Work out the finished part from the listing and answer in its coordinate system (mm). Face numbers are marked on the shaded views. A direction names the side the tool comes from. Round coordinates to 2 decimals unless told otherwise and drop trailing zeros. Write each loop counter-clockwise with the first axis right and the second up, starting at its lowest first coordinate (ties: lowest second). Pieces come first, ordered by that corner, then holes. Notation, with made-up numbers: M -18.75,17 L 37.25,17 A19 cw 37.25,49 Z; hole C 42.25,64.5 d2. An arc over 180 degrees is marked long. One line per item, written item: value. Start each with the question number.
Q1. A tool of negligible diameter and unlimited length cuts with its end or side. For the marked faces 1, 2, 3 and 4, from which of +Z, -Z, +X, -X, +Y, -Y can it reach the whole face along a straight path? Write none if from no direction.
Q2. Find section C-C (x = 15). Write down the section's boundary in (y, z).
Q3. The mould has two halves that part along X. Classify the marked faces 5, 6, 7 and 8: released by +X, released by -X, zero draft, split by the parting line, or undercut.
Q4. Find section A-A (z = 0). Write down the section's boundary in (x, y), and give its area (4 significant figures).
Q5. Find section D-D (z = -12.5). Write down the section's boundary in (x, y), and give its area (3 significant figures).
Q6. Given pin 1 Ø1 at (y, z) = (4, -18.5) entering from +X; pin 2 Ø1 at (y, z) = (8.5, -14) entering from -X; pin 3 Ø0.6 at (x, y) = (7.5, 2) entering from +Z, each flat-ended and moving along its own axis, determine where each tip first touches the part or whether it passes through.
Q7. Consider probe 1 along X at (y, z) = (1.8, 0); probe 2 along Z at (x, y) = (14.25, 1.5); probe 3 along Y at (x, z) = (3.25, -3). Determine where each line is inside the solid, lowest interval first.
Q8. Find section B-B (y = 4.25). Write down the section's boundary in (x, z).
from build123d import *

# Parameters (mm, degrees)
MAIN_BODY_DEPTH                           = 10
SKETCH1_3_R                               = 1.6
CONNECTOR_BODY_DEPTH                      = 5
DULLING_FILLET_START                      = 5
DULLING_FILLET_DEPTH                      = 6
CUT_EXTRUDE1_DEPTH                        = 45.806187552
FILLET1_R                                 = 2
FILLET2_R                                 = 0.5
ELEPHANTSFOOT_COMPENSATION_LEFT_CONF_SIZE = 0.5


with BuildPart() as part:
    # complete_sketch → main_body (new body)
    with BuildSketch(Plane(origin=(0, 0, 0), x_dir=(1, 0, 0), z_dir=(0, 1, 0))):
        with BuildLine():
            ThreePointArc((-2.5, 8.291561976), (-2.925728922, 5.40481063), (-4.166666667, 2.763853992))
            ThreePointArc((-4.166666667, 2.763853992), (-1.24767584, 4.841828683), (2.312045751, 4.433333333))
            ThreePointArc((2.312045751, 4.433333333), (4.555661111, 3.587465144), (6.936137254, 3.3))
            Line((6.936137254, 3.3), (8.063862746, 3.3))
            ThreePointArc((8.063862746, 3.3), (10.444338889, 3.587465144), (12.687954249, 4.433333333))
            ThreePointArc((12.687954249, 4.433333333), (16.605433979, 4.735248857), (19.531538935, 2.113091309))
            Line((19.531538935, 2.113091309), (3.218923361, 37.095608299))
            ThreePointArc((3.218923361, 37.095608299), (-0.149318842, 38.756641535), (-2.5, 35.827753514))
            Line((-2.5, 35.827753514), (-2.5, 8.291561976))
        make_face()
    extrude(amount=MAIN_BODY_DEPTH)

    # Sketch1<3> → connector_body (add)
    with BuildSketch(Plane(origin=(0, 0, 0), x_dir=(1, 0, 0), z_dir=(0, 1, 0))):
        with BuildLine():
            ThreePointArc((2.312045751, -4.433333333), (4.555661111, -3.587465144), (6.936137254, -3.3))
            Line((6.936137254, -3.3), (8.063862746, -3.3))
            ThreePointArc((8.063862746, -3.3), (10.444338889, -3.587465144), (12.687954249, -4.433333333))
            ThreePointArc((12.687954249, -4.433333333), (18.456219958, -3.613107195), (19.531538935, 2.113091309))
            ThreePointArc((19.531538935, 2.113091309), (16.605433979, 4.735248857), (12.687954249, 4.433333333))
            ThreePointArc((12.687954249, 4.433333333), (10.444338889, 3.587465144), (8.063862746, 3.3))
            Line((8.063862746, 3.3), (6.936137254, 3.3))
            ThreePointArc((6.936137254, 3.3), (4.555661111, 3.587465144), (2.312045751, 4.433333333))
            ThreePointArc((2.312045751, 4.433333333), (-1.24767584, 4.841828683), (-4.166666667, 2.763853992))
            ThreePointArc((-4.166666667, 2.763853992), (-3.716151374, -3.345178466), (2.312045751, -4.433333333))
        make_face()
        with Locations(Location((0, 0, 0), (0, 0, 270))):
            Circle(SKETCH1_3_R, mode=Mode.SUBTRACT)
        with Locations(Location((15, 0, 0), (0, 0, 270))):
            Circle(SKETCH1_3_R, mode=Mode.SUBTRACT)
    extrude(amount=CONNECTOR_BODY_DEPTH)

    # dulling_fillet: read off the stored shape, not the designer's step
    # dulling_fillet outline → dulling_fillet (cut)
    with BuildSketch(Plane(origin=(0, 0, 0), x_dir=(1, 0, 0), z_dir=(0, 1, 0)).offset(DULLING_FILLET_START)):
        with BuildLine():
            Line((19.531538935, 2.113091309), (18.195102647, 4.979088177))
            ThreePointArc((18.195102647, 4.979088177), (18.080055144, 4.399425861), (17.492680685, 4.334344587))
            ThreePointArc((17.492680685, 4.334344587), (18.683531845, 3.381063908), (19.531538935, 2.113091309))
        make_face()
        with BuildLine():
            ThreePointArc((-4.166666667, 2.763853992), (-3.358016887, 3.704554303), (-2.342670216, 4.417227214))
            ThreePointArc((-2.342670216, 4.417227214), (-2.902133749, 4.479151002), (-3.049464036, 5.022407651))
            ThreePointArc((-3.049464036, 5.022407651), (-3.536643042, 3.85780149), (-4.166666667, 2.763853992))
        make_face()
    extrude(amount=DULLING_FILLET_DEPTH, mode=Mode.SUBTRACT)

    # Sketch2 → Cut-Extrude1 (cut, through all)
    with BuildSketch(Plane(origin=(0, 10, 0), x_dir=(1, 0, 0), z_dir=(0, 1, 0))):
        Polygon((-2.5, 8.291561976), (-0.068911087, 6.887972137), (0.531088913, 7.927202622), (-2.5, 9.677202622), align=None)
        Polygon((4.275469015, 34.829838831), (2.267951488, 31.962806676), (3.250933941, 31.274514953), (4.861066057, 33.574021924), align=None)
    extrude(amount=-CUT_EXTRUDE1_DEPTH, mode=Mode.SUBTRACT)

    # Fillet1
    fillet1_edges = [part.edges().sort_by_distance(p)[0] for p in [
        (-2.5, 5, -9.677202622),
        (4.275469015, 5, -34.829838831),
    ]]
    fillet(fillet1_edges, radius=FILLET1_R)

    # Fillet2
    fillet2_edges = [part.edges().sort_by_distance(p)[0] for p in [
        (4.861066057, 5, -33.574021924),
        (-2.5, 5, -8.291561976),
    ]]
    fillet(fillet2_edges, radius=FILLET2_R)

    # elephantsfoot_compensation_left_conf
    elephantsfoot_compensation_left_conf_edges = [part.edges().sort_by_distance(p)[0] for p in [
        (-0.484455543, 0, -8.513527487),
        (0.231088913, 0, -7.40758738),
        (3.807634117, 0, -32.069565198),
        (2.759442715, 0, -31.618660815),
        (-2.5, 0, -23.329828337),
        (-0.149318842, 0, -38.756641535),
        (2.940555742, 0, -32.923385101),
        (3.503197421, 0, -36.48598061),
        (-2.232050808, 0, -9.83190316),
        (12.379301571, 0, -17.451113833),
        (3.967245303, 0, -34.856804912),
        (-3.049950658, 0, -5.021001256),
        (-0.926536362, 0, -7.383122321),
        (-2.266493544, 0, -7.888003391),
        (4.817488185, 0, -33.075924575),
        (-3.716151374, 0, 3.345178466),
        (18.456219958, 0, 3.613107195),
        (7.5, 0, 3.3),
        (10.444338889, 0, 3.587465144),
        (0, 0, -1.6),
        (15, 0, -1.6),
        (4.555661111, 0, 3.587465144),
    ]]
    chamfer(elephantsfoot_compensation_left_conf_edges, length=ELEPHANTSFOOT_COMPENSATION_LEFT_CONF_SIZE)


solid = part.part
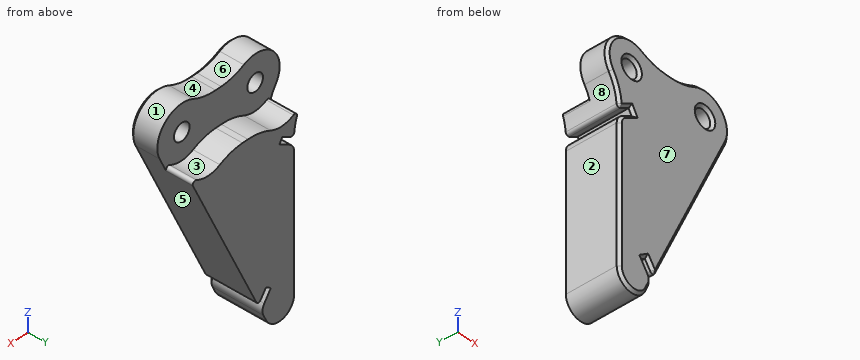
The answers:
1. face 1: +Y, -Y
1. face 2: -Z, -X, +Y, -Y
1. face 3: +Z, +Y
1. face 4: +Z, +Y, -Y
2. outline: M 0,-10.65 L 0.5,-11.83 L 10,-11.83 L 10,-5 L 5,-5 L 5,-1.6 L 0.5,-1.6 L 0,-2.1 Z; M 0,2.1 L 0.5,1.6 L 5,1.6 L 5,5 L 0.5,5 L 0,4.5 Z
3. face 5: released by +X
3. face 6: undercut
3. face 7: zero draft
3. face 8: released by -X
4. outline: M -5,0.5 L -4.5,0 L -2.1,0 L -1.6,0.5 L -1.6,5 L -5,5 Z; M 1.6,0.5 L 2.1,0 L 12.9,0 L 13.4,0.5 L 13.4,5 L 1.6,5 Z; M 16.6,0.5 L 17.1,0 L 19.5,0 L 20,0.5 L 20,5 L 16.6,5 Z
4. area: 92.25 mm2
5. outline: M -2.5,0.5 L -2,0 L 14.14,0 L 14.69,0.5 L 14.69,10 L -2.5,10 Z
5. area: 172 mm2
6. pin 1: x = 12.12
6. pin 2: x = -2.5
6. pin 3: z = 3.3
7. probe 1: -5 to -1.6, 1.6 to 13.4, 16.6 to 20
7. probe 2: -13.44 to -1.41, 1.41 to 4.94
7. probe 3: 0 to 5
8. outline: M -4.17,-2.76 A10 cw -2.53,-7.49 A0.5 ccw -1.78,-7.88 L -0.07,-6.89 L 0.53,-7.93 L -1.5,-9.1 A2 ccw -2.5,-10.83 L -2.5,-35.83 A3 ccw 3.22,-37.1 L 3.79,-35.88 A2 ccw 3.61,-33.88 L 2.27,-31.96 L 3.25,-31.27 L 4.36,-32.86 A0.5 ccw 5.23,-32.79 L 19.53,-2.11 A5 ccw 12.69,4.43 A10 cw 8.06,3.3 L 6.94,3.3 A10 cw 2.31,4.43 A5 ccw Z; hole C 0,0 d3.2; hole C 15,0 d3.2
